Part model, mm, in its own coordinate system. Face numbers are marked on the shaded views. Give positions to 0.01 mm unless a question says otherwise; leave off trailing zeros. Order: outer loops, then holes, each group sorted by start corner. A loop starts at its lowest first (then second) coordinate and runs counter-clockwise, first axis right, second up.
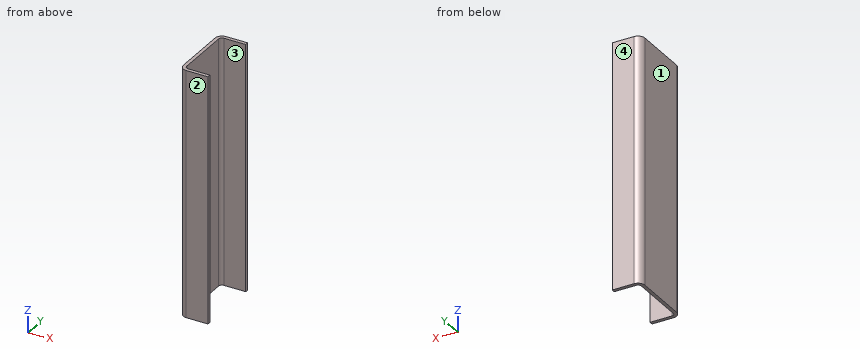
from build123d import *

# Parameters (mm, degrees)
SKETCH1_W                      = 228.6
SKETCH1_H                      = 63.5
BASE_FLANGE1_DEPTH             = 3.175
EDGE_FLANGE1_STRIP_W           = 19.05
EDGE_FLANGE1_STRIP_H           = 3.175
EDGE_FLANGE1_STRIP_CUT_DEPTH   = 228.6
EDGE_FLANGE1_STRIP_2_W         = 19.05
EDGE_FLANGE1_STRIP_2_H         = 3.175
EDGE_FLANGE1_STRIP_CUT_2_DEPTH = 228.6
EDGE_FLANGE1_DEPTH             = 228.6
EDGE_FLANGE1_BEND_DEPTH        = 228.6


# Sheet-metal steps are written as plain solids
with BuildPart() as part:
    # Sketch1 → Base-Flange1 (new body)
    with BuildSketch(Plane(origin=(0, 0, 0), x_dir=(0, 0, -1), z_dir=(1, 0, 0))):
        with Locations((114.3, 31.75)):
            Rectangle(SKETCH1_W, SKETCH1_H)
    extrude(amount=-BASE_FLANGE1_DEPTH)

    # Edge-Flange1 strip (across the edge) → Edge-Flange1 strip cut (cut)
    with BuildSketch(Plane(origin=(0, 63.5, -228.6), x_dir=(0, -1, 0), z_dir=(0, 0, 1))):
        with Locations((-3.175, -1.5875)):
            Rectangle(EDGE_FLANGE1_STRIP_W, EDGE_FLANGE1_STRIP_H)
    extrude(amount=EDGE_FLANGE1_STRIP_CUT_DEPTH, mode=Mode.SUBTRACT)

    # Edge-Flange1 strip 2 (across the edge) → Edge-Flange1 strip cut 2 (cut)
    with BuildSketch(Plane.YX):
        with Locations((-3.175, -1.5875)):
            Rectangle(EDGE_FLANGE1_STRIP_2_W, EDGE_FLANGE1_STRIP_2_H)
    extrude(amount=EDGE_FLANGE1_STRIP_CUT_2_DEPTH, mode=Mode.SUBTRACT)

    # Edge-Flange1 section (across the edge) → Edge-Flange1 (add)
    with BuildSketch(Plane(origin=(0, 63.5, -228.6), x_dir=(0, -1, 0), z_dir=(0, 0, 1))):
        with BuildLine():
            Line((0, 3.175), (0, 23.368))
            Line((0, 23.368), (3.175, 23.368))
            Line((3.175, 23.368), (3.175, 3.175))
            ThreePointArc((3.175, 3.175), (4.10493597, 0.92993597), (6.35, 0))
            Line((6.35, 0), (6.35, -3.175))
            ThreePointArc((6.35, -3.175), (1.859871939, -1.315128061), (0, 3.175))
        make_face()
    extrude(amount=EDGE_FLANGE1_DEPTH)

    # Edge-Flange1 section 2 (across the edge) → Edge-Flange1 bend (add)
    with BuildSketch(Plane.YX):
        with BuildLine():
            Line((0, 3.175), (0, 23.368))
            Line((0, 23.368), (3.175, 23.368))
            Line((3.175, 23.368), (3.175, 3.175))
            ThreePointArc((3.175, 3.175), (4.10493597, 0.92993597), (6.35, 0))
            Line((6.35, 0), (6.35, -3.175))
            ThreePointArc((6.35, -3.175), (1.859871939, -1.315128061), (0, 3.175))
        make_face()
    extrude(amount=EDGE_FLANGE1_BEND_DEPTH)


solid = part.part
Item 1: Band-saw the part on B-B on z = -26. List the corners of the cut face in (x, y) (3 decimals).
Item 2: Band-saw the part on A-A on x = 8.5. List the corners of the cut face in (y, z) (3 decimals), plus the area to 3 significant figures.
Item 3: Drop a flat-ended pin along its axis: P1, Ø1.5, axis at y = 29, z = -84, coming from the +X side. Give the stop position or say it passes through.
Item 4: Band-saw the part on C-C on y = 11. List the corners of the cut face in (x, z) (3 decimals).
Item 5: Pull direction Y, two halves, no side cores. Call the marked faces 1, 2, 3 and 4: released by +Y, released by -Y, zero draft, split by the parting line, or undercut.
Item 6: Drill centre lines: probe 1 along Y at (x, z) = (14.25, -182.5) (3 decimals); probe 2 along X at (y, z) = (57, -213) (3 decimals); probe 3 along Y at (x, z) = (2.25, -164.5). Where is each one in solid material? Low to high.
Working result:
1. outline: (-3.175, 6.35) arc R6.35 ccw to (3.175, 0) - (23.368, 0) - (23.368, 3.175) - (3.175, 3.175) arc R3.175 cw to (0, 6.35) - (0, 57.15) arc R3.175 cw to (3.175, 60.325) - (23.368, 60.325) - (23.368, 63.5) - (3.175, 63.5) arc R6.35 ccw to (-3.175, 57.15) - close
2. outline: (0, -228.6) - (3.175, -228.6) - (3.175, 0) - (0, 0) - close; (60.325, -228.6) - (63.5, -228.6) - (63.5, 0) - (60.325, 0) - close
2. area: 1,450 mm2
3. P1: stops at x = 0
4. outline: (-3.175, -228.6) - (0, -228.6) - (0, 0) - (-3.175, 0) - close
5. face 1: zero draft
5. face 2: released by -Y
5. face 3: undercut
5. face 4: released by +Y
6. probe 1: y = 0 to 3.175, 60.325 to 63.5
6. probe 2: x = -3.175 to 0
6. probe 3: y = 0.07 to 3.31, 60.19 to 63.43
